```python
from build123d import *

# Parameters (mm, degrees)
F0_W      = 29.3
F0_H      = 31
F1_DEPTH  = 3
F2_W      = 6
F2_H      = 3
F5_DEPTH  = 21.65
F3_W      = 6
F3_H      = 3
F6_DEPTH  = 21.65
F4_W      = 6
F4_H      = 3
F7_DEPTH  = 22.65
F8_W      = 4
F8_H      = 6
F8_W_2    = 6
F8_H_2    = 4
F9_DEPTH  = 24
F10_W     = 6
F10_H     = 4
F13_DEPTH = 35.95
F11_W     = 6
F11_H     = 4
F14_DEPTH = 35.95
F12_W     = 6
F12_H     = 4
F15_DEPTH = 33.8
F17_DEPTH = 4
F19_DEPTH = 3
F21_DEPTH = 10


with BuildPart() as f1:
    # F0 (on Top) → F1 (new body)
    with BuildSketch(Plane.XY):
        with Locations((-17.4727943537, 14.6659919992)):
            Rectangle(F0_W, F0_H)
    extrude(amount=F1_DEPTH)

    # F2 (on face) → F5 (join)
    with BuildSketch(Plane.YZ.offset(-2.8227943537)):
        with Locations((14.6659919992, 1.5)):
            Rectangle(F2_W, F2_H)
    extrude(amount=F5_DEPTH)

    # F3 (on face) → F6 (join)
    with BuildSketch(Plane(origin=(-32.1227943537, 0, 0), x_dir=(0, -1, 0), z_dir=(-1, 0, 0))):
        with Locations((-14.6659919992, 1.5)):
            Rectangle(F3_W, F3_H)
    extrude(amount=F6_DEPTH)

    # F4 (on face) → F7 (join)
    with BuildSketch(Plane.XZ.offset(0.8340080008)):
        with Locations((-17.4727943537, 1.5)):
            Rectangle(F4_W, F4_H)
    extrude(amount=F7_DEPTH)

    # F8 (on face) → F9 (join)
    with BuildSketch(Plane.XY.offset(3)):
        with Locations((16.8272056463, 14.6659919992)):
            Rectangle(F8_W, F8_H)
        with Locations((-17.4727943537, -21.4840080008)):
            Rectangle(F8_W_2, F8_H_2)
        with Locations((-51.7727943537, 14.6659919992)):
            Rectangle(F8_W, F8_H)
    extrude(amount=F9_DEPTH)

    # F10 (on face) → F13 (join)
    with BuildSketch(Plane(origin=(14.8272056463, 0, 0), x_dir=(0, -1, 0), z_dir=(-1, 0, 0))):
        with Locations((-14.6659919992, 25)):
            Rectangle(F10_W, F10_H)
    extrude(amount=F13_DEPTH)

    # F11 (on face) → F14 (join)
    with BuildSketch(Plane.YZ.offset(-49.7727943537)):
        with Locations((14.6659919992, 25)):
            Rectangle(F11_W, F11_H)
    extrude(amount=F14_DEPTH)

    # F12 (on face) → F15 (join)
    with BuildSketch(Plane(origin=(0, -19.4840080008, 0), x_dir=(-1, 0, 0), z_dir=(0, 1, 0))):
        with Locations((17.4727943537, 25)):
            Rectangle(F12_W, F12_H)
    extrude(amount=F15_DEPTH)

    # F16 (on face) → F17 (cut)
    with BuildSketch(Plane.XY.offset(3)):
        with BuildLine():
            ThreePointArc((-17.4727943537, 13.6659919992), (-16.7656875725, 13.958885218), (-16.4727943537, 14.6659919992))
            Line((-16.4727943537, 14.6659919992), (-17.4727943537, 14.6659919992))
            Line((-17.4727943537, 14.6659919992), (-17.4727943537, 13.6659919992))
        make_face()
        with BuildLine():
            Line((-17.4727943537, 14.6659919992), (-16.4727943537, 14.6659919992))
            ThreePointArc((-16.4727943537, 14.6659919992), (-16.7656875725, 15.3730987804), (-17.4727943537, 15.6659919992))
            Line((-17.4727943537, 15.6659919992), (-17.4727943537, 14.6659919992))
        make_face()
        with BuildLine():
            Line((-18.4727943537, 14.6659919992), (-17.4727943537, 14.6659919992))
            Line((-17.4727943537, 14.6659919992), (-17.4727943537, 15.6659919992))
            ThreePointArc((-17.4727943537, 15.6659919992), (-18.1799011348, 15.3730987804), (-18.4727943537, 14.6659919992))
        make_face()
        with BuildLine():
            Line((-17.4727943537, 13.6659919992), (-17.4727943537, 14.6659919992))
            Line((-17.4727943537, 14.6659919992), (-18.4727943537, 14.6659919992))
            ThreePointArc((-18.4727943537, 14.6659919992), (-18.1799011348, 13.958885218), (-17.4727943537, 13.6659919992))
        make_face()
    extrude(amount=-F17_DEPTH, mode=Mode.SUBTRACT)

    # F18 (on face) → F19 (join)
    with BuildSketch(Plane.XY.offset(27)):
        Polygon((-14.4727943537, -17.4840080008), (-14.4727943537, -23.4840080008), (18.8272056463, -23.4840080008), (18.8272056463, 11.6659919992), (12.8272056463, 11.6659919992), (12.8272056463, -17.4840080008), align=None)
        Polygon((-47.7727943537, 11.6659919992), (-53.7727943537, 11.6659919992), (-53.7727943537, -23.4840080008), (-20.4727943537, -23.4840080008), (-20.4727943537, -17.4840080008), (-47.7727943537, -17.4840080008), align=None)
    extrude(amount=-F19_DEPTH)

    # F20 (on face) → F21 (join)
    with BuildSketch(Plane.XZ.offset(23.4840080008)):
        Polygon((-53.7727943537, 24), (-20.4727943537, 24), (-14.4727943537, 24), (18.8272056463, 24), (18.8272056463, 27), (-53.7727943537, 27), align=None)
    extrude(amount=F21_DEPTH)


solid = f1.part
```
Model file for the job. Use its own axes, mm. A direction names the side the tool comes from. Round coordinates to 2 decimals unless told otherwise and drop trailing zeros. Write each loop counter-clockwise with the first axis right and the second up, starting at its lowest first coordinate (ties: lowest second). Pieces come first, ordered by that corner, then holes. Notation, with made-up numbers: (52, -30.75) - (59, -30.75) arc R27 ccw to (59, -8.75) - close; hole circle Ø6 at (38.5, 12.25). An arc over 180 degrees is marked (long way). One line per item, written item: value.
(1) Cut at D-D, the plane y = 22.5. Give the cut face in (x, z), plus the area to 3 significant figures.
Values follow:
outline: (-32.12, 0) - (-2.82, 0) - (-2.82, 3) - (-32.12, 3) - close
area: 87.9 mm²
(2) Cut at A-A, the plane x = -35.5. Give the cut face in (y, z).
Values follow:
outline: (-33.48, 24) - (-17.48, 24) - (-17.48, 27) - (-33.48, 27) - close; (11.67, 0) - (17.67, 0) - (17.67, 3) - (11.67, 3) - close; (11.67, 23) - (17.67, 23) - (17.67, 27) - (11.67, 27) - close
(3) Wall check: probe 1 along Z at (x, y) = (7, 13); probe 2 along X at (y, z) = (12, 15.5); probe 3 along Y at (x, z) = (-11, 24.5). Give the ranges that are in metal, low to high.
Values follow:
probe 1: z = 0 to 3, 23 to 27
probe 2: x = -53.77 to -49.77, 14.83 to 18.83
probe 3: y = -33.48 to -17.48, 11.67 to 17.67
(4) Drop flat-ended pins along their axis: P1, Ø3, axis at x = -17.5, z = 19, coming from the -Y side; P2, Ø8, axis at x = -22.5, z = 9.5, coming from the +Y side; P3, Ø2.5, axis at x = -3, z = 25.5, coming from the +Y side. Give the stop position or say it passes through.
Values follow:
P1: stops at y = -23.48
P2: stops at y = -19.48
P3: stops at y = 17.67
(5) 3-axis set-ups, long thin cutter, end or side, ignore diameter. For faces 4 (the flat face through (-34, -17.484, 26)), 5 (the flat face through (-17, 9, 23)), 6 (the flat face through (-42.1, 11.666, 23.4)), 7 (the flat face through (-18, -19.484, 13)), 8 (the flat face through (-49.773, 15, 13)): which of +Z, -Z, +X, -X, +Y, -Y reach the whole face in a straight line?
Values follow:
face 4: +Z, -Z
face 5: +Y
face 6: none
face 7: +X, -X, +Y
face 8: +Y, -Y
(6) Cut at C-C, the plane y = -5. Give the cut face in (x, z).
Values follow:
outline: (-53.77, 24) - (-47.77, 24) - (-47.77, 27) - (-53.77, 27) - close; (-20.47, 0) - (-14.47, 0) - (-14.47, 3) - (-20.47, 3) - close; (-20.47, 23) - (-14.47, 23) - (-14.47, 27) - (-20.47, 27) - close; (12.83, 24) - (18.83, 24) - (18.83, 27) - (12.83, 27) - close
(7) Cut at B-B, the plane z = 6. Give the cut face in (x, y).
Values follow:
outline: (-53.77, 11.67) - (-49.77, 11.67) - (-49.77, 17.67) - (-53.77, 17.67) - close; (-20.47, -23.48) - (-14.47, -23.48) - (-14.47, -19.48) - (-20.47, -19.48) - close; (14.83, 11.67) - (18.83, 11.67) - (18.83, 17.67) - (14.83, 17.67) - close
(8) Two-plate mould, pull along Y, no slides. Class faces 1 (the flat face through (-32.123, 24, 1)), 2 (the flat face through (-26, -0.834, 1)), 3 (the flat face through (7, 11.666, 23.4)): pulls with the +Y half, pulls with the -Y half, needs draft (parallel to the pull), parting line crosses it, or undercut.
Values follow:
face 1: needs draft
face 2: pulls with the -Y half
face 3: undercut
